The listing builds one solid part. Answer for the finished solid, in the listing's coordinates (mm). Face numbers are marked on the shaded views. A direction names the side the tool comes from. Give positions to 0.01 mm unless a question says otherwise; leave off trailing zeros. Order: outer loops, then holes, each group sorted by start corner. A loop starts at its lowest first (then second) coordinate and runs counter-clockwise, first axis right, second up. Notation, with made-up numbers: (-7, 57.5) - (1, 57.5) arc R27 cw to (1, 81.5) - close; hole circle Ø2 at (35.5, 13.5). An arc over 180 degrees is marked (long way). Answer as a JSON object with one key per item and string values. Group by question number.
Q1. A cutting plane is placed at D-D, the plane z = 22. Give the vertices of the cut face in (x, y), and give its area (3 significant figures).
Q2. The mould has two halves that part along Z. Classify the marked faces 5, 6 and 7: released by +Z, released by -Z, zero draft, split by the parting line, or undercut.
Q3. A cutting plane is placed at C-C, the plane x = 1.5. Give the vertices of the cut face in (y, z), and give its area (3 significant figures).
Q4. A cutting plane is placed at B-B, the plane z = 62. Give the vertices of the cut face in (x, y), and give its area (3 significant figures).
Q5. Given pin 1 (11 mm diameter, centred on x = 17, y = -12, fed in from +Z); pin 2 (12 mm diameter, centred on y = 13.5, z = 22.5, fed in from +X); pin 3 (12.5 mm diameter, centred on x = 8.5, z = 47, fed in from -Y), each flat-ended and moving along its own axis, determine where each tip first touches the part or whether it passes through.
Q6. A cutting plane is placed at A-A, the plane x = 18. Give the vertices of the cut face in (y, z), and give its area (3 significant figures).
Q7. For the marked faces 1, 2, 3 and 4, determine the directions among +Z, -Z, +X, -X, +Y, -Y from which every point of the face is accessible in a straight line to the end or side of a thin tool.
Q8. Consider line 1 (Y direction, x = 9, z = 9); line 2 (X direction, y = 15, z = 69.5); line 3 (Z direction, x = -0.5, y = -8.5). Determine where each line is inside the solid, lowest interval first.
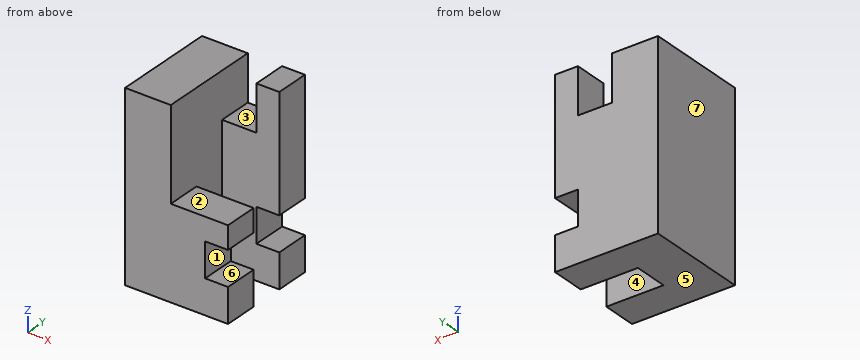
from build123d import *

# Parameters (mm, degrees)
F0_W     = 45
F0_H     = 45
F1_DEPTH = 80
F4_DEPTH = 80
F3_W     = 15
F3_H     = 20
F3_W_2   = 10
F3_H_2   = 15
F5_DEPTH = 45
F6_W     = 25
F6_H     = 15
F7_DEPTH = 40
F8_DEPTH = 40


with BuildPart() as f1:
    # F0 (on Top) → F1 (new body)
    with BuildSketch(Plane.XY):
        Rectangle(F0_W, F0_H)
    extrude(amount=F1_DEPTH)

    # F2 (on face) → F4 (cut)
    with BuildSketch(Plane.XY.offset(80)):
        Polygon((22.5, -7.5), (22.5, 7.5), (12.5, 7.5), (-2.5, 7.5), (-2.5, -7.5), (12.5, -7.5), align=None)
    extrude(amount=-F4_DEPTH, mode=Mode.SUBTRACT)

    # F3 (on face) → F5 (cut)
    with BuildSketch(Plane.XZ.offset(22.5)):
        with Locations((5, 70)):
            Rectangle(F3_W, F3_H)
        with Locations((17.5, 22.5)):
            Rectangle(F3_W_2, F3_H_2)
    extrude(amount=-F5_DEPTH, mode=Mode.SUBTRACT)

    # F6 (on face) → F7 (cut)
    with BuildSketch(Plane.XY.offset(80)):
        with Locations((10, -15)):
            Rectangle(F6_W, F6_H)
    extrude(amount=-F7_DEPTH, mode=Mode.SUBTRACT)

    # F6 (on face) → F8 (cut)
    with BuildSketch(Plane.XY.offset(80)):
        with Locations((10, -15)):
            Rectangle(F6_W, F6_H)
    extrude(amount=-F8_DEPTH, mode=Mode.SUBTRACT)


solid = f1.part
Reply:
{
 "1": {"outline": "(-22.5, -22.5) - (12.5, -22.5) - (12.5, -7.5) - (-2.5, -7.5) - (-2.5, 7.5) - (12.5, 7.5) - (12.5, 22.5) - (-22.5, 22.5) - close", "area": "1,350 mm^2"},
 "2": {"face 5": "released by -Z", "face 6": "undercut", "face 7": "zero draft"},
 "3": {"outline": "(-22.5, 0) - (-7.5, 0) - (-7.5, 40) - (-22.5, 40) - close; (7.5, 0) - (22.5, 0) - (22.5, 60) - (7.5, 60) - close", "area": "1,500 mm^2"},
 "4": {"outline": "(-22.5, -22.5) - (-2.5, -22.5) - (-2.5, 22.5) - (-22.5, 22.5) - close; (12.5, 7.5) - (22.5, 7.5) - (22.5, 22.5) - (12.5, 22.5) - close", "area": "1,050 mm^2"},
 "5": {"pin 1": "stops at z = 40", "pin 2": "stops at x = 12.5", "pin 3": "stops at y = 7.5"},
 "6": {"outline": "(-22.5, 0) - (-7.5, 0) - (-7.5, 15) - (-22.5, 15) - close; (-22.5, 30) - (-7.5, 30) - (-7.5, 40) - (-22.5, 40) - close; (7.5, 0) - (22.5, 0) - (22.5, 15) - (7.5, 15) - close; (7.5, 30) - (22.5, 30) - (22.5, 80) - (7.5, 80) - close", "area": "1,350 mm^2"},
 "7": {"face 1": "+X, +Y, -Y", "face 2": "+Z, +X, -Y", "face 3": "+Z, +Y, -Y", "face 4": "+Z, -Z, +X"},
 "8": {"line 1": "y = -22.5 to -7.5, 7.5 to 22.5", "line 2": "x = -22.5 to -2.5, 12.5 to 22.5", "line 3": "z = 0 to 40"}
}
